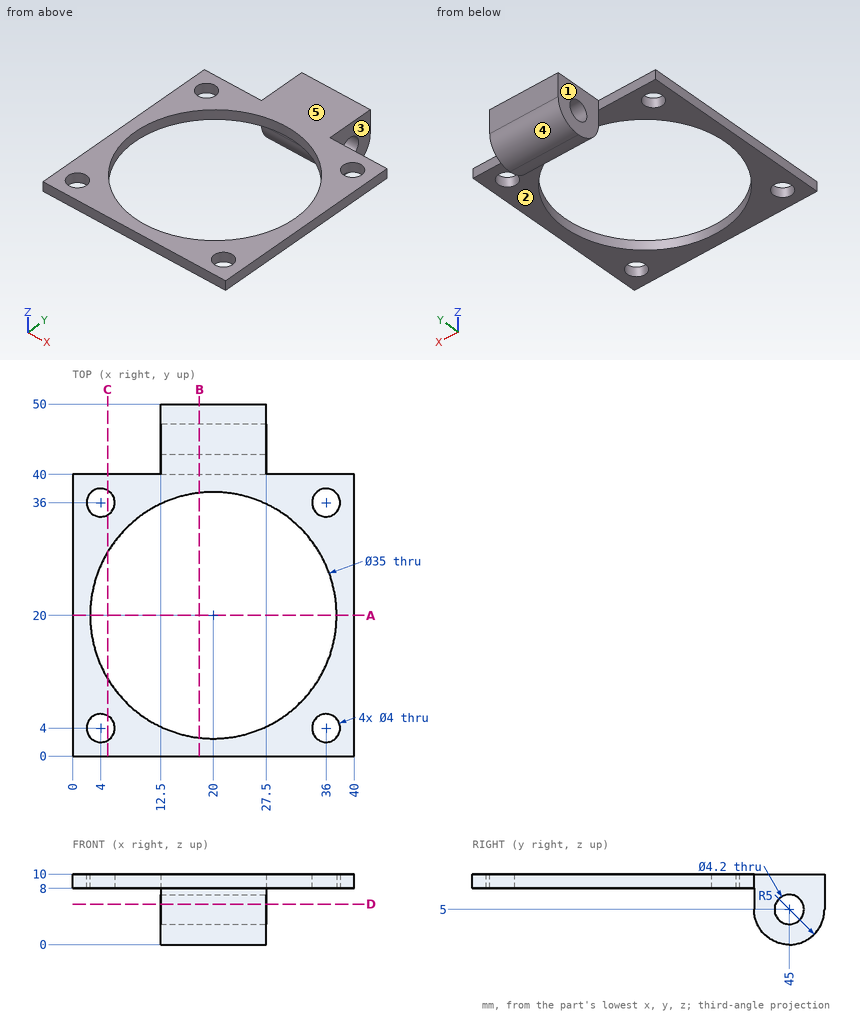
The figure shows three views and two pictorial views of one solid part (mm, origin at its lowest corner). Answer the questions. A direction names the side the tool comes from. Round coordinates to 2 decimals unless told otherwise and drop trailing zeros. Order: outer loops, then holes, each group sorted by start corner. A loop starts at its lowest first (then second) coordinate and runs counter-clockwise, first axis right, second up. Notation, with made-up numbers: (30, 49.5) -> (57, 49.5) arc R11 cw to (57, 57.5) -> close; hole circle Ø5 at (75.25, 76). An arc over 180 degrees is marked (long way). One line per item, written item: value.
Item 1: Find section D-D, the plane z = 5.75. Give the vertices of the cut face in (x, y).
Taken from the geometry:
outline: (12.5, 40) -> (27.5, 40) -> (27.5, 43.04) -> (12.5, 43.04) -> close; (12.5, 46.96) -> (27.5, 46.96) -> (27.5, 50) -> (12.5, 50) -> close
Item 2: Find section B-B, the plane x = 18. State how many separate pieces and enclosed holes the cut face has, then the cut area to 3 significant figures.
Taken from the geometry:
separate pieces: 2
enclosed holes: 1
area: 85.9 mm2
Item 3: Find section C-C, the plane x = 5. Give the vertices of the cut face in (y, z), then the cut area to 3 significant figures.
Taken from the geometry:
outline: (0, 8) -> (2.27, 8) -> (2.27, 10) -> (0, 10) -> close; (5.73, 8) -> (10.99, 8) -> (10.99, 10) -> (5.73, 10) -> close; (29.01, 8) -> (34.27, 8) -> (34.27, 10) -> (29.01, 10) -> close; (37.73, 8) -> (40, 8) -> (40, 10) -> (37.73, 10) -> close
area: 30.1 mm2
Item 4: Given P1, Ø1.5, axis at x = 16.5, y = 40, coming from the -Z side; P2, Ø1.5, axis at x = 19, z = 6, coming from the -Y side; P3, Ø5, axis at x = 32.5, y = 29, coming from the -Z side, each flat-ended and moving along its own axis, determine where each tip first touches the part or whether it passes through.
Taken from the geometry:
P1: stops at z = 2.37
P2: stops at y = 40
P3: stops at z = 8
Item 5: Straight lines are drawn through the part: L1, parallel to Y at x = 4, z = 9.05; L2, parallel to X at y = 5.5, z = 9.25; L3, parallel to X at y = 46, z = 1.5. For each, find the intervals that lie inside material, in ascending order.
Taken from the geometry:
L1: y = 0 to 2, 6 to 12.91, 27.09 to 34, 38 to 40
L2: x = 0 to 2.68, 5.32 to 10.2, 29.8 to 34.68, 37.32 to 40
L3: x = 12.5 to 27.5
Item 6: For the marked faces 1, 2, 3, 4 and 5, determine the directions among +Z, -Z, +X, -X, +Y, -Y from which every point of the face is accessible in a straight line to the end or side of a thin tool.
Taken from the geometry:
face 1: +Z, -Z, -X, +Y
face 2: -Z, +X, -X, -Y
face 3: +Z, -Z, +X, +Y
face 4: -Z, +X, -X, +Y
face 5: +Z, +X, -X, +Y, -Y
Item 7: Find section A-A, the plane y = 20. Give the vertices of the cut face in (x, z), then the cut area to 3 significant figures.
Taken from the geometry:
outline: (0, 8) -> (2.5, 8) -> (2.5, 10) -> (0, 10) -> close; (37.5, 8) -> (40, 8) -> (40, 10) -> (37.5, 10) -> close
area: 10.0 mm2
